```python
from build123d import *

# Parameters (mm, degrees)
SCHIZZO1_W                   = 68
SCHIZZO1_H                   = 40
ESTRUSIONE_ESTRUSIONE1_DEPTH = 26
SCHIZZO2_R                   = 5
TAGLIO_ESTRUSIONE1_DEPTH     = 84.066238629
SCHIZZO3_R                   = 2.5
TAGLIO_ESTRUSIONE2_DEPTH     = 84.066238629


with BuildPart() as part:
    # Schizzo1 → Estrusione-Estrusione1 (new body)
    with BuildSketch(Plane.XY):
        with Locations((34, 20)):
            Rectangle(SCHIZZO1_W, SCHIZZO1_H)
    extrude(amount=-ESTRUSIONE_ESTRUSIONE1_DEPTH)

    # Schizzo2 → Taglio-Estrusione1 (cut, through all)
    with BuildSketch(Plane.ZY):
        with Locations(Location((-13, 20, 0), (0, 0, 270))):
            Circle(SCHIZZO2_R)
    extrude(amount=-TAGLIO_ESTRUSIONE1_DEPTH, mode=Mode.SUBTRACT)

    # Schizzo3 → Taglio-Estrusione2 (cut, through all)
    with BuildSketch(Plane(origin=(0, 0, -26), x_dir=(-1, 0, 0), z_dir=(0, 0, -1))):
        with Locations((-11, 34)):
            Circle(SCHIZZO3_R)
        with Locations((-57, 34)):
            Circle(SCHIZZO3_R)
        with Locations((-57, 6)):
            Circle(SCHIZZO3_R)
        with Locations((-11, 6)):
            Circle(SCHIZZO3_R)
    extrude(amount=-TAGLIO_ESTRUSIONE2_DEPTH, mode=Mode.SUBTRACT)


solid = part.part
```
Verification items for the finished model (mm, model axes). Give positions to 0.01 mm unless a question says otherwise; leave off trailing zeros. Order: outer loops, then holes, each group sorted by start corner. A loop starts at its lowest first (then second) coordinate and runs counter-clockwise, first axis right, second up. Notation, with made-up numbers: M 18.5,41.25 L 66.5,41.25 A18 cw 66.5,67.25 Z; hole C 46.5,50.25 d8. An arc over 180 degrees is marked long. Answer in a Markdown table with one row per item. Add a question column.
Item 1: Scan lines: probe 1 along Y at (x, z) = (11, -6.5); probe 2 along Y at (x, z) = (57, -15.75); probe 3 along Z at (x, y) = (16, 20). Record each from-to range of solid material in increasing order. Write a range as from..to.
Item 2: Section check B-B, the plane x = 11. Enter the section's corners in (y, z).
Item 3: Gauge pin test, flat end, axial feed: pin 1 (3 mm diameter, centred on x = 11, y = 6, fed in from -Z) (3 decimals). Record the tip position at first contact, or that the pin passes through.
Item 4: Section check C-C, the plane y = 6. Enter the section's corners in (x, z), and give its area (3 significant figures).
Item 5: Section check D-D, the plane y = 20. Enter the section's corners in (x, z).
Item 6: Mould release check, pull along X, two halves, no side actions. Record for faces 1 (the cylindrical face through (12.84, 35.69, -13.18)), 2 (the flat face through (34, 20, 0)), 3 (the flat face through (68, 15, -10)): released by +X, released by -X, zero draft, split by the parting line, or undercut.
Item 7: Section check A-A, the plane z = -13. Enter the section's corners in (x, y).
Filled sheet:
| question | item | result |
|---|---|---|
| 1 | probe 1 | y = 0..3.5, 8.5..31.5, 36.5..40 |
| 1 | probe 2 | y = 0..3.5, 8.5..15.82, 24.18..31.5, 36.5..40 |
| 1 | probe 3 | z = -26..-18, -8..0 |
| 2 | outline | M 0,-26 L 3.5,-26 L 3.5,0 L 0,0 Z; M 8.5,-26 L 31.5,-26 L 31.5,0 L 8.5,0 Z; M 36.5,-26 L 40,-26 L 40,0 L 36.5,0 Z; hole C 20,-13 d10 |
| 3 | pin 1 | passes through |
| 4 | outline | M 0,-26 L 8.5,-26 L 8.5,0 L 0,0 Z; M 13.5,-26 L 54.5,-26 L 54.5,0 L 13.5,0 Z; M 59.5,-26 L 68,-26 L 68,0 L 59.5,0 Z |
| 4 | area | 1,510 mm^2 |
| 5 | outline | M 0,-26 L 68,-26 L 68,-18 L 0,-18 Z; M 0,-8 L 68,-8 L 68,0 L 0,0 Z |
| 6 | face 1 | undercut |
| 6 | face 2 | zero draft |
| 6 | face 3 | released by +X |
| 7 | outline | M 0,0 L 68,0 L 68,15 L 0,15 Z; M 0,25 L 68,25 L 68,40 L 0,40 Z; hole C 11,6 d5; hole C 11,34 d5; hole C 57,6 d5; hole C 57,34 d5 |
